Work out the finished part from the listing and answer in its coordinate system (mm). A direction names the side the tool comes from. Coordinates: 2 decimals unless noted, no trailing zeros. Order: outer loops, then holes, each group sorted by start corner. A loop starts at its lowest first (then second) coordinate and runs counter-clockwise, first axis right, second up.
1. The part is cut by section C-C, the plane z = -1.1. Give the vertices of the cut face in (x, y), then the cut area to 4 significant figures.
2. Determine the mould class of faces 4 (the flat face through (0, 0, 2.5)), 5 (the flat face through (0, -1.25, 0)), 6 (the flat face through (-3.75, 0, 0)) for opening direction X: +X half, -X half, draft (parallel to the pull), parting line (faces both ways), or undercut.
3. Flat-ended cylindrical pins translate along their axes: pin 1 Ø2 at (y, z) = (0, 1) entering from -X; pin 2 Ø0.8 at (y, z) = (0, 0.5) entering from +X; pin 3 Ø0.7 at (x, z) = (4, 3) entering from +Y. Find the tip coordinate at first contact, or state that the pin passes through.
4. The part is cut by section B-B, the plane y = 0.5. Give the vertices of the cut face in (x, z).
5. The part is cut by section D-D, the plane y = 1. Give the vertices of the cut face in (x, z), then the cut area to 3 significant figures.
6. Find the intervals of material crossed by probe 1 along Z at (x, y) = (2.75, -1.1); probe 2 along Y at (x, z) = (0.5, 1.05); probe 3 along X at (y, z) = (-0.1, -0.1), in increasing order.
7. A tool of negligible diameter and unlimited length cuts with its end or side. For faces 1 (the flat face through (3.479, -0.011, 2.796)), 2 (the flat face through (3.75, 0, 0)), 3 (the flat face through (0, 1.25, 0)), from which of +Z, -Z, +X, -X, +Y, -Y can it reach the whole face along a straight path? Write none if from no direction.
8. The part is cut by section A-A, the plane x = 1. Give the vertices of the cut face in (y, z).
```python
from build123d import *

# Parameters (mm, degrees)
BOSS_EXTRUDE1_DEPTH      = 1.25
BOSS_EXTRUDE1_DEPTH_BACK = 1.25
SKETCH1_W                = 7.5
SKETCH1_H                = 5
BOSS_EXTRUDE2_DEPTH      = 0.8
BOSS_EXTRUDE2_DEPTH_BACK = 0.8
BOSS_EXTRUDE3_DEPTH      = 2.5
BOSS_EXTRUDE3_DEPTH_BACK = 2.5


with BuildPart() as part:
    # Sketch1 → Boss-Extrude1 (new, two sides: drawn at the far end of the back side and taken through both)
    with BuildSketch(Plane(origin=(0, 0, 0), x_dir=(1, 0, 0), z_dir=(0, 1, 0)).offset(-BOSS_EXTRUDE1_DEPTH_BACK)):
        Rectangle(SKETCH1_W, SKETCH1_H)
    extrude(amount=BOSS_EXTRUDE1_DEPTH + BOSS_EXTRUDE1_DEPTH_BACK)

    # Sketch3 → Boss-Extrude2 (add, two sides: drawn at the far end of the back side and taken through both)
    with BuildSketch(Plane(origin=(0, 0, 0), x_dir=(1, 0, 0), z_dir=(0, 1, 0)).offset(-BOSS_EXTRUDE2_DEPTH_BACK)):
        Polygon((-3.75, -2.5), (-4.3, -2.752945266), (-4.14038936, -3.1), (-2.835759292, -2.5), align=None)
        Polygon((3.75, -2.5), (2.835759292, -2.5), (4.14038936, -3.1), (4.3, -2.752945266), align=None)
    extrude(amount=BOSS_EXTRUDE2_DEPTH + BOSS_EXTRUDE2_DEPTH_BACK)

    # Sketch5 → Boss-Extrude3 (add, two sides: drawn at the far end of the back side and taken through both)
    with BuildSketch(Plane(origin=(0, 0, 0), x_dir=(0, 0, -1), z_dir=(1, 0, 0)).offset(-BOSS_EXTRUDE3_DEPTH_BACK)):
        Polygon((-2.5, 1.25), (-3.1, 1.8), (-3.1, 1.350797038), (-2.5, 0.800797038), align=None)
        Polygon((-2.5, -0.800797038), (-2.5, -1.25), (-3.1, -1.8), (-3.1, -1.350797038), align=None)
    extrude(amount=BOSS_EXTRUDE3_DEPTH + BOSS_EXTRUDE3_DEPTH_BACK)


solid = part.part
```
Geometry says:
1. outline: (-3.75, -1.25) - (3.75, -1.25) - (3.75, 1.25) - (-3.75, 1.25) - close
1. area: 18.75 mm2
2. face 4: undercut
2. face 5: draft
2. face 6: -X half
3. pin 1: stops at x = -3.75
3. pin 2: stops at x = 3.75
3. pin 3: stops at y = 0.8
4. outline: (-4.3, 2.75) - (-3.75, 2.5) - (-3.75, -2.5) - (3.75, -2.5) - (3.75, 2.5) - (4.3, 2.75) - (4.14, 3.1) - (2.84, 2.5) - (-2.84, 2.5) - (-4.14, 3.1) - close
5. outline: (-3.75, -2.5) - (3.75, -2.5) - (3.75, 2.5) - (2.5, 2.5) - (2.5, 2.72) - (-2.5, 2.72) - (-2.5, 2.5) - (-3.75, 2.5) - close
5. area: 38.6 mm2
6. probe 1: z = -2.5 to 2.5
6. probe 2: y = -1.25 to 1.25
6. probe 3: x = -3.75 to 3.75
7. face 1: +Z, +Y, -Y
7. face 2: -Z, +X, +Y, -Y
7. face 3: -Z, +X, -X, +Y
8. outline: (-1.8, 3.1) - (-1.25, 2.5) - (-1.25, -2.5) - (1.25, -2.5) - (1.25, 2.5) - (1.8, 3.1) - (1.35, 3.1) - (0.8, 2.5) - (-0.8, 2.5) - (-1.35, 3.1) - close
